The model under review builds one solid part; all positions refer to its coordinate system, in mm. A direction names the side the tool comes from. Round coordinates to 2 decimals unless told otherwise and drop trailing zeros. Order: outer loops, then holes, each group sorted by start corner. A loop starts at its lowest first (then second) coordinate and runs counter-clockwise, first axis right, second up.
1) Consider section B-B (z = -103). Give the boundary of the cut face in (x, y).
2) Consider section C-C (y = 35). Give the boundary of the cut face in (x, z), then the cut area to 3 significant figures.
3) Consider section D-D (z = -43). Give the number of separate pieces and of enclosed holes in the cut face, then the cut area to 3 significant figures.
4) Machinability: for faces 5 (the face through (-31.908, 3.944, -17.601)), 6 (the face through (-4, 35, -49)), which of the approach directions +Z, -Z, +X, -X, +Y, -Y give a long, thin tool a straight path to every point of the face, cutting with its end or side? Answer none if there is none.
5) Clearance check with a flat-ended pin moving along its axis: P1, Ø3.5, axis at x = -30, z = -103, coming from the -Y side. State where the tip first meets the part, or that it passes through.
6) Mouldability with a two-part tool opening along X and no side actions: class faces 1 (the face through (-28.092, 86.944, -16.399)), 2 (the face through (0, 45, -61)), 3 (the face through (-4, 33, -25)), 4 (the face through (-20, 4, -79)) as pulls with the +X half, pulls with the -X half, needs draft (parallel to the pull), parting line crosses it, or undercut.
7) Consider section A-A (x = -6.5). Give the boundary of the cut face in (y, z).
8) To check wall thickness, follow L1, parallel to Y at x = -14, z = -21; L2, parallel to Y at x = -3.75, z = -60; L3, parallel to X at y = 32, z = -64. State the ranges of each line that lie inside material, in increasing order.
Autodesk Inventor part; units mm, degrees
ref_plane "Work Plane1" through (0, 83, 0) normal (0, -1, 0) x (1, 0, 0)
ref_plane "YZ Plane" through (0, 0, 0) normal (1, 0, 0) x (0, 1, 0)
ref_plane "XZ Plane" through (0, 0, 0) normal (0, 1, 0) x (-1, 0, 0)
sketch "Sketch1" plane through (0, 0, 0) normal (0, 1, 0) x (-1, 0, 0)
  line L0 (0, 0) -> (8, 0)
  line L1 (8, 0) -> (8, -120)
  line L2 (8, -120) -> (0, -120)
  line L3 (0, -120) -> (0, 0)
  line L4 (8, 0) -> (38, 0)
  line L5 (38, 0) -> (38, -120)
  line L6 (38, -120) -> (8, -120)
  line L7 (8, -120) -> (8, 0)
  circle A0 centre (20, -17) radius 2
  circle A1 centre (20, -30) radius 2
  circle A2 centre (20, -43) radius 2
  circle A3 centre (20, -77) radius 2
  circle A4 centre (20, -90) radius 2
  circle A5 centre (20, -103) radius 2
  circle A6 centre (30, -17) radius 2
  circle A7 centre (30, -30) radius 2
  circle A8 centre (30, -43) radius 2
  circle A9 centre (30, -77) radius 2
  circle A10 centre (30, -90) radius 2
  circle A11 centre (30, -103) radius 2
  dimension "d15" = 8
  dimension "d16" = 120
  dimension "d17" = 30
extrude "Extrusion3" add sketch "Sketch1" along normal blind 83 contours L0 L1 L2 L3
extrude "Extrusion4" add sketch "Sketch1" along normal blind 8 contours L4 L5 L6 L1
sketch "Sketch2" plane through (0, 0, 0) normal (1, 0, 0) x (0, 0, -1)
  line L0 (0, 0) -> (120, 0)
  line L1 (120, 0) -> (120, 83)
  line L2 (0, 0) -> (0, 35)
  line L3 (0, 8) -> (0, 83)
  circle A0 centre (25, 35) radius 2
  circle A1 centre (60, 35) radius 2
  dimension "d53" = 4
  dimension "d54" = 4
extrude "Extrusion5" cut sketch "Sketch2" against normal blind 10
ref_plane "Work Plane1" through (0, 83, 0) normal (0, -1, 0) x (1, 0, 0)
sketch "Sketch4" plane through (0, 83, 0) normal (0, -1, 0) x (1, 0, 0)
  line L0 (0, -120) -> (0, 0)
  line L1 (0, 0) -> (-8, 0)
  line L2 (-8, 0) -> (-8, -120)
  line L3 (-8, -120) -> (0, -120)
  line L4 (-8, 0) -> (-38, 0)
  line L5 (-38, 0) -> (-38, -120)
  line L6 (-38, -120) -> (-8, -120)
  line L7 (-8, -120) -> (-8, 0)
  circle A0 centre (-20, -17) radius 2
  circle A1 centre (-20, -30) radius 2
  circle A2 centre (-20, -43) radius 2
  circle A3 centre (-20, -77) radius 2
  circle A4 centre (-20, -90) radius 2
  circle A5 centre (-20, -103) radius 2
  circle A6 centre (-30, -77) radius 2
  circle A7 centre (-30, -90) radius 2
  circle A8 centre (-30, -103) radius 2
  circle A9 centre (-30, -43) radius 2
  circle A10 centre (-30, -30) radius 2
  circle A11 centre (-30, -17) radius 2
  point P0 (8, -120)
extrude "Extrusion6" add sketch "Sketch4" against normal blind 8
fillet "Fillet1" radius 4 6 edges at (-38, 87, 0) (-38, 87, -120) (-38, 4, -120) (-38, 4, 0) (-8, 83, -60) (-8, 8, -60)
sketch "Sketch5" plane through (-8, 12, 0) normal (-1, 0, 0) x (0, 0, 1)
  circle A0 centre (-60, 23) radius 2
  circle A1 centre (-25, 23) radius 2
  line L0 (-49, 23) -> (-49, 35)
  line L1 (-49, 35) -> (-30, 35)
  line L2 (-30, 35) -> (-30, 23)
  line L3 (-30, 23) -> (-30, 11)
  line L4 (-30, 11) -> (-49, 11)
  line L5 (-49, 11) -> (-49, 23)
  point P0 (0, -12)
extrude "Extrusion7" cut sketch "Sketch5" against normal blind 10 contours L0 L1 L2 L3 L4 L5
sketch "Sketch6" plane through (-8, 12, 0) normal (-1, 0, 0) x (0, 0, 1)
  line L0 (-116, -12) -> (-4, -12)
  line L1 (-116, 79) -> (-4, 79)
  line L2 (-27, 23) -> (-23, 23)
  circle A0 centre (-25, 23) radius 2
  point P0 (0, -12)
  dimension "d57" = 91
  dimension "d58" = 35
  dimension "d59" = 56
properties part number "_3DPrint"
Answer below:
1. outline: (-38, 0) - (-32, 0) - (-32, 8) - (-38, 8) - close; (-38, 83) - (-32, 83) - (-32, 91) - (-38, 91) - close; (-28, 0) - (-22, 0) - (-22, 8) - (-28, 8) - close; (-28, 83) - (-22, 83) - (-22, 91) - (-28, 91) - close; (-18, 0) - (0, 0) - (0, 91) - (-18, 91) - (-18, 83) - (-12, 83) arc R4 cw to (-8, 79) - (-8, 12) arc R4 cw to (-12, 8) - (-18, 8) - close
2. outline: (-8, -120) - (0, -120) - (0, -62) - (-8, -62) - close; (-8, -58) - (0, -58) - (0, -49) - (-8, -49) - close; (-8, -30) - (0, -30) - (0, -27) - (-8, -27) - close; (-8, -23) - (0, -23) - (0, 0) - (-8, 0) - close
2. area: 744 mm2
3. separate pieces: 6
3. enclosed holes: 0
3. area: 895 mm2
4. face 5: +Y, -Y
4. face 6: +X, -X
5. P1: passes through
6. face 1: undercut
6. face 2: pulls with the +X half
6. face 3: needs draft
6. face 4: undercut
7. outline: (0, -120) - (91, -120) - (91, 0) - (0, 0) - close; hole (23, -49) - (47, -49) - (47, -30) - (23, -30) - close; hole circle Ø4 at (35, -60); hole circle Ø4 at (35, -25)
8. L1: y = 0 to 8, 83 to 91
8. L2: y = 0 to 33, 37 to 91
8. L3: x = -8 to 0
